from build123d import *

# Parameters (mm, degrees)
SKETCH1_W                = 80
SKETCH1_H                = 39
BOSS_EXTRUDE1_DEPTH      = 10
BOSS_EXTRUDE2_START      = -12.5
SKETCH4_R                = 8
SKETCH4_R_2              = 6
BOSS_EXTRUDE2_DEPTH      = 24.5
SKETCH10_W               = 22.023984498
SKETCH10_H               = 20.291265962
BOSS_EXTRUDE4_DEPTH      = 10
SKETCH13_W               = 3
SKETCH13_H               = 20
BOSS_EXTRUDE5_DEPTH      = 20
SKETCH14_R               = 5
CUT_EXTRUDE1_DEPTH       = 15
BOSS_EXTRUDE6_DEPTH      = 10
BOSS_EXTRUDE6_DEPTH_BACK = 10
SKETCH16_R               = 6.726812024
SKETCH16_R_2             = 4.5
FILLET2_R                = 4
FILLET4_R                = 2
FILLET8_R                = 10
FILLET9_R                = 8
FILLET15_R               = 4
FILLET16_R               = 2


with BuildPart() as part:
    # Sketch1 → Boss-Extrude1 (new body)
    with BuildSketch(Plane(origin=(0, 0, 0), x_dir=(1, 0, 0), z_dir=(0, 1, 0))):
        Polygon((11.011992249, 112.28929502), (75, 49), (75, -6), (50, -6), (50, 0), (-50, 0), (-50, -6), (-75, -6), (-75, 49), (-11.011992249, 112.28929502), align=None)
        with Locations((0, 29.5)):
            Rectangle(SKETCH1_W, SKETCH1_H, mode=Mode.SUBTRACT)
    extrude(amount=BOSS_EXTRUDE1_DEPTH)

    # Sketch4 → Boss-Extrude2 (add)
    with BuildSketch(Plane(origin=(-62.5, 0, 0), x_dir=(0, 0, -1), z_dir=(1, 0, 0)).offset(BOSS_EXTRUDE2_START)):
        with Locations((-12, 5)):
            Circle(SKETCH4_R)
        with Locations((-12, 5)):
            Circle(SKETCH4_R_2, mode=Mode.SUBTRACT)
    boss_extrude2 = extrude(amount=BOSS_EXTRUDE2_DEPTH)

    # Mirror1: Boss-Extrude2 across plane
    add(boss_extrude2.mirror(Plane(origin=(0, 0, 0), x_dir=(0, 0, 1), z_dir=(1, 0, 0))))

    # Sketch10 → Boss-Extrude4 (add)
    with BuildSketch(Plane(origin=(0, 10, 0), x_dir=(1, 0, 0), z_dir=(0, 1, 0))):
        with Locations((0, 122.434928001)):
            Rectangle(SKETCH10_W, SKETCH10_H)
    extrude(amount=-BOSS_EXTRUDE4_DEPTH)

    # Sketch13 → Boss-Extrude5 (add)
    with BuildSketch(Plane(origin=(0, 10, 0), x_dir=(1, 0, 0), z_dir=(0, 1, 0))):
        with Locations((-4, 94.28929502)):
            Rectangle(SKETCH13_W, SKETCH13_H)
        with Locations((4, 94.28929502)):
            Rectangle(SKETCH13_W, SKETCH13_H)
    extrude(amount=BOSS_EXTRUDE5_DEPTH)

    # Sketch14 → Cut-Extrude1 (cut)
    with BuildSketch(Plane(origin=(5.5, 0, 0), x_dir=(0, 0, -1), z_dir=(1, 0, 0))):
        with Locations((94.28929502, 22)):
            Circle(SKETCH14_R)
    extrude(amount=-CUT_EXTRUDE1_DEPTH, mode=Mode.SUBTRACT)

    # Sketch16 → Boss-Extrude6 (add, two sides: drawn at the far end of the back side and taken through both)
    with BuildSketch(Plane(origin=(0, 0, 0), x_dir=(0, 0, -1), z_dir=(1, 0, 0)).offset(-BOSS_EXTRUDE6_DEPTH_BACK)):
        with Locations((137.080560982, 5)):
            Circle(SKETCH16_R)
        with Locations(Location((137.080560982, 5, 0), (0, 0, 180))):
            Circle(SKETCH16_R_2, mode=Mode.SUBTRACT)
    extrude(amount=BOSS_EXTRUDE6_DEPTH + BOSS_EXTRUDE6_DEPTH_BACK)

    # Fillet2
    fillet2_edges = [part.edges().sort_by_distance(p)[0] for p in [
        (-4, 10, -104.28929502),
        (-5.5, 10, -94.28929502),
        (-4, 10, -84.28929502),
    ]]
    fillet(fillet2_edges, radius=FILLET2_R)

    # Fillet4
    fillet4_edges = [part.edges().sort_by_distance(p)[0] for p in [
        (40, 0, -29.5),
        (0, 0, -49),
        (-40, 0, -29.5),
        (0, 0, -10),
        (40, 5, -10),
        (40, 5, -49),
        (-40, 5, -49),
        (-40, 5, -10),
        (0, 10, -10),
        (-40, 10, -29.5),
        (0, 10, -49),
        (40, 10, -29.5),
    ]]
    fillet(fillet4_edges, radius=FILLET4_R)

    # Fillet8
    fillet8_edges = [part.edges().sort_by_distance(p)[0] for p in [
        (11.011992249, 5, -112.28929502),
        (75, 5, -49),
        (-75, 5, -49),
        (-11.011992249, 5, -112.28929502),
        (-62.75, 0, 5.755002002),
        (-62.75, 10, 5.755002002),
        (62.75, 0, 5.755002002),
        (62.75, 10, 5.755002002),
    ]]
    fillet(fillet8_edges, radius=FILLET8_R)

    # Fillet9
    # the kernel refuses this fillet: 8 mm, written as the material it adds along each edge
    with BuildSketch(Plane(origin=(10, 5, -132.580560982), x_dir=(1, 0, 0), z_dir=(0, -1, 0))) as fillet9_piece_1_section:
        with BuildLine():
            CenterArc((8, -3.894579268), FILLET9_R, 150.868059199, 29.131940801)
            Line((0, -3.894579268), (0, 0))
            Line((0, 0), (1.011992249, 0))
        make_face()
    fillet9_piece_1 = extrude(amount=14.73644817, mode=Mode.PRIVATE)
    fillet9_piece_1 = fillet9_piece_1 - Plane(origin=(10, 5, -137.080560982), x_dir=(0, 0, 1), z_dir=(-1, 0, 0)) * Cylinder(4.5, 46, mode=Mode.PRIVATE)
    fillet9_piece_1 = fillet9_piece_1 & Plane(origin=(10, 5, -137.080560982), x_dir=(0, 0, -1), z_dir=(-1, 0, 0)) * Cylinder(6.726812024, 46, mode=Mode.PRIVATE)
    add(fillet9_piece_1)
    with BuildSketch(Plane(origin=(10, 19.73644817, -132.580560982), x_dir=(1, 0, 0), z_dir=(0, -1, 0))) as fillet9_piece_2_section:
        with BuildLine():
            CenterArc((8, -3.894579268), FILLET9_R, 150.868059199, 29.131940801)
            Line((0, -3.894579268), (0, 0))
            Line((0, 0), (1.011992249, 0))
        make_face()
    fillet9_piece_2 = extrude(amount=14.73644817, mode=Mode.PRIVATE)
    fillet9_piece_2 = fillet9_piece_2 - Plane(origin=(10, 5, -137.080560982), x_dir=(0, 0, 1), z_dir=(-1, 0, 0)) * Cylinder(4.5, 46, mode=Mode.PRIVATE)
    fillet9_piece_2 = fillet9_piece_2 & Plane(origin=(10, 5, -137.080560982), x_dir=(0, 0, -1), z_dir=(-1, 0, 0)) * Cylinder(6.726812024, 46, mode=Mode.PRIVATE)
    add(fillet9_piece_2)
    with BuildSketch(Plane(origin=(-10, 5, -132.580560982), x_dir=(0, 0, -1), z_dir=(0, -1, 0))) as fillet9_piece_3_section:
        with BuildLine():
            CenterArc((3.894579268, -8), FILLET9_R, 90, 29.131940801)
            Line((0, -1.011992249), (0, 0))
            Line((0, 0), (3.894579268, 0))
        make_face()
    fillet9_piece_3 = extrude(amount=14.73644817, mode=Mode.PRIVATE)
    fillet9_piece_3 = fillet9_piece_3 - Plane(origin=(-10, 5, -137.080560982), x_dir=(0, 0, 1), z_dir=(-1, 0, 0)) * Cylinder(4.5, 46, mode=Mode.PRIVATE)
    fillet9_piece_3 = fillet9_piece_3 & Plane(origin=(-10, 5, -137.080560982), x_dir=(0, 0, -1), z_dir=(-1, 0, 0)) * Cylinder(6.726812024, 46, mode=Mode.PRIVATE)
    add(fillet9_piece_3)
    with BuildSketch(Plane(origin=(-10, 19.73644817, -132.580560982), x_dir=(0, 0, -1), z_dir=(0, -1, 0))) as fillet9_piece_4_section:
        with BuildLine():
            CenterArc((3.894579268, -8), FILLET9_R, 90, 29.131940801)
            Line((0, -1.011992249), (0, 0))
            Line((0, 0), (3.894579268, 0))
        make_face()
    fillet9_piece_4 = extrude(amount=14.73644817, mode=Mode.PRIVATE)
    fillet9_piece_4 = fillet9_piece_4 - Plane(origin=(-10, 5, -137.080560982), x_dir=(0, 0, 1), z_dir=(-1, 0, 0)) * Cylinder(4.5, 46, mode=Mode.PRIVATE)
    fillet9_piece_4 = fillet9_piece_4 & Plane(origin=(-10, 5, -137.080560982), x_dir=(0, 0, -1), z_dir=(-1, 0, 0)) * Cylinder(6.726812024, 46, mode=Mode.PRIVATE)
    add(fillet9_piece_4)

    # Fillet15
    fillet15_edges = [part.edges().sort_by_distance(p)[0] for p in [
        (5.5, 10, -94.28929502),
        (4, 10, -104.28929502),
        (4, 10, -84.28929502),
    ]]
    fillet(fillet15_edges, radius=FILLET15_R)

    # Fillet16
    fillet16_edges = [part.edges().sort_by_distance(p)[0] for p in [
        (2.5, 10, -94.28929502),
        (-2.5, 10, -94.28929502),
    ]]
    fillet(fillet16_edges, radius=FILLET16_R)


solid = part.part
Check sheet for the modelled part. Datum: model origin and axes. Units: mm. A direction names the side the tool comes from. Round coordinates to 2 decimals unless told otherwise and drop trailing zeros. Loops run counter-clockwise (first coordinate to the right, second up) from the corner with the lowest first, then second, coordinate; pieces in that order, holes last. Notation, with made-up numbers: M 80,11.25 L 93,11.25 A13 cw 93,16.25 Z; hole C 29,5 d6. An arc over 180 degrees is marked long. One line per question, with ' | ' between items. Start each with the question number.
Item 1: Set-up check for faces 1 (the face through (10, 5, -142)), 2 (the face through (-1, 5, -10)), 3 (the face through (50, 5, 3)), 4 (the face through (2.5, 17, -96)), 5 (the face through (6.703, 11.141, -94.485)): record each of +Z, -Z, +X, -X, +Y, -Y from which the full face is reachable in a straight line by a thin tool's end or side.
Item 2: Release check for a two-part mould opening along Z. For faces 6 (the face through (62.92, -0.44, 4.98)), 7 (the face through (-10, 5, -142)), 8 (the face through (-3.979, 20.085, -98.908)) record: released by +Z, released by -Z, zero draft, split by the parting line, or undercut.
Item 3: Gauge pin test, flat ends, axial feed: pin 1 Ø6 at (y, z) = (7, -65) entering from +X; pin 2 Ø0.9 at (x, y) = (-3.5, 24.5) entering from +Z; pin 3 Ø3 at (x, y) = (18, 5) entering from +Z. Record the tip position at first contact, or that the pin passes through.
Item 4: Section check C-C (z = -24). Record the boundary of the cut face in (x, y).
Item 5: Scan lines: probe 1 along Z at (x, y) = (4, 5.5); probe 2 along Y at (x, z) = (58.5, 12); probe 3 along X at (y, z) = (23, -104). Record each from-to range of solid material in increasing order.
Item 6: Section check B-B (y = 22). Record the boundary of the cut face in (x, z), and give its area (3 significant figures).
Item 7: Section check A-A (z = 12). Record the boundary of the cut face in (x, y), and give its area (3 significant figures).
Item 8: Section check D-D (x = -63). Record the boundary of the cut face in (y, z).
Worked out:
1) face 1: -Z, +X, +Y, -Y | face 2: +Y, -Y | face 3: +Z, +Y, -Y | face 4: +Z, -Z, +Y | face 5: +Z, +X, +Y
2) face 6: released by -Z | face 7: zero draft | face 8: undercut
3) pin 1: x = 61.86 | pin 2: z = -84.29 | pin 3: z = 0
4) outline: M -75,0 L -42,0 A2 ccw -40,2 L -40,8 A2 ccw -42,10 L -75,10 Z; M 40,2 A2 ccw 42,0 L 75,0 L 75,10 L 42,10 A2 ccw 40,8 Z
5) probe 1: -143.79 to -141.55, -132.61 to -49, -10 to 0 | probe 2: -3 to -1, 11 to 13 | probe 3: -5.5 to -2.5, 2.5 to 5.5
6) outline: M -5.5,-104.29 L -2.5,-104.29 L -2.5,-99.29 L -5.5,-99.29 Z; M -5.5,-89.29 L -2.5,-89.29 L -2.5,-84.29 L -5.5,-84.29 Z; M 2.5,-104.29 L 5.5,-104.29 L 5.5,-99.29 L 2.5,-99.29 Z; M 2.5,-89.29 L 5.5,-89.29 L 5.5,-84.29 L 2.5,-84.29 Z | area: 60.0 mm^2
7) outline: M -75,-3 L -50.5,-3 L -50.5,-1 L -75,-1 Z; M -75,11 L -50.5,11 L -50.5,13 L -75,13 Z; M 50.5,-3 L 75,-3 L 75,-1 L 50.5,-1 Z; M 50.5,11 L 75,11 L 75,13 L 50.5,13 Z | area: 196 mm^2
8) outline: M -1.67,7.58 A10 cw 0,2.05 L 0,-60.87 L 10,-60.87 L 10,2.05 A10 cw 11.67,7.58 A8 ccw long Z; hole C 5,12 d12
